For this review, use the dimensioned drawing (mm, ordinates from the lowest corner) and the shaded views. A direction names the side the tool comes from. Coordinates: 2 decimals unless noted, no trailing zeros. Write each loop counter-clockwise with the first axis right and the second up, starting at its lowest first coordinate (ties: lowest second). Pieces come first, ordered by that corner, then holes. Notation, with made-up numbers: (-1, -32.5) - (37, -32.5) arc R37 cw to (37, 5.5) - close; hole circle Ø3 at (-28.75, 53). An arc over 180 degrees is marked (long way). Put each result on its own line as item: value.
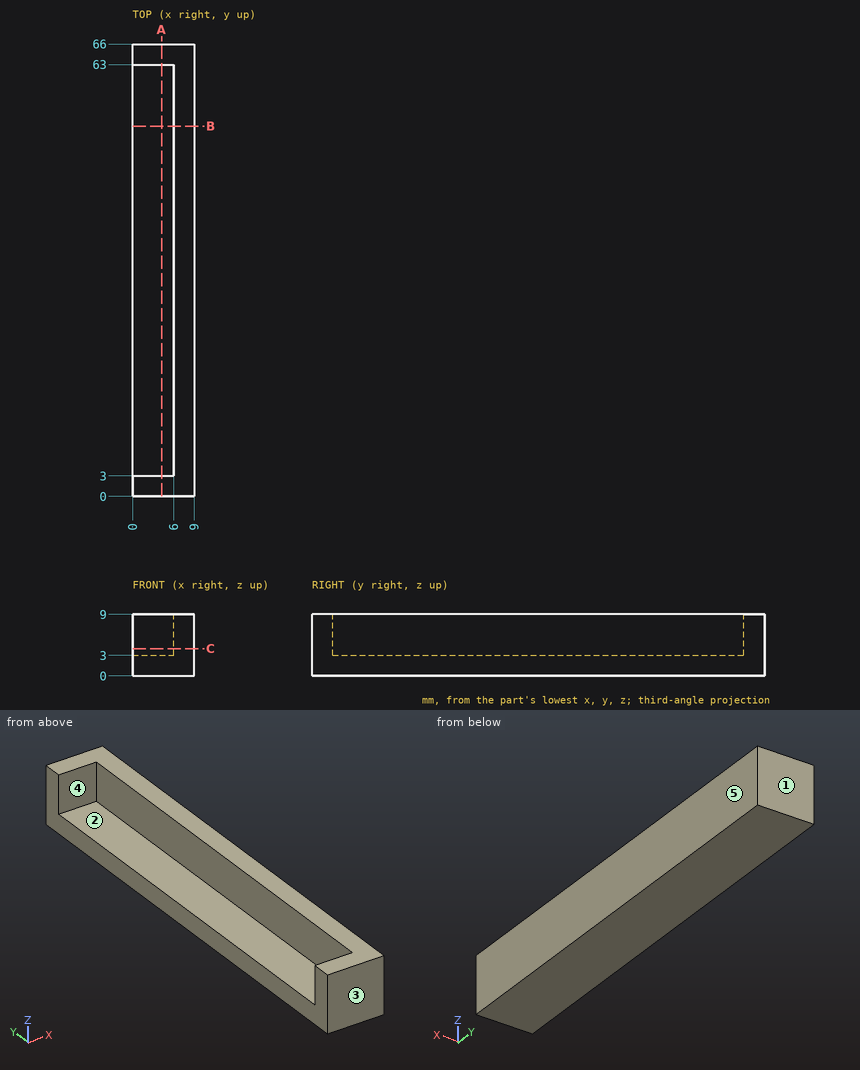
1. Machinability: for the marked faces 4 and 5, which of the approach directions +Z, -Z, +X, -X, +Y, -Y give a long, thin tool a straight path to every point of the face, cutting with its end or side? Answer none if there is none.
Determined:
face 4: +Z, -X
face 5: +Z, -Z, +X, +Y, -Y
2. The part is to be moulded in two halves that separate along Y. For the marked faces 1, 2 and 3, say which applies: +Y half, -Y half, draft (parallel to the pull), parting line (faces both ways), or undercut.
Determined:
face 1: +Y half
face 2: undercut
face 3: -Y half
3. Consider section B-B on y = 54. State the section outline as (x, z) points, plus the area to 3 significant figures.
Determined:
outline: (0, 0) - (9, 0) - (9, 9) - (6, 9) - (6, 3) - (0, 3) - close
area: 45.0 mm^2
4. For pin 1 Ø1.8 at (y, z) = (19, 6.5) entering from -X; pin 2 Ø5 at (x, y) = (2.5, 34.5) entering from +Z, all flat-tipped, find the tip position at first contact; note any pin that passes through.
Determined:
pin 1: stops at x = 6
pin 2: stops at z = 3
5. Consider section A-A on x = 4.25. State the section outline as (y, z) points, plus the area to 3 significant figures.
Determined:
outline: (0, 0) - (66, 0) - (66, 9) - (63, 9) - (63, 3) - (3, 3) - (3, 9) - (0, 9) - close
area: 234 mm^2
6. To check wall thickness, follow probe 1 along Y at (x, z) = (2.25, 3.25); probe 2 along X at (y, z) = (47, 4.5); probe 3 along Z at (x, y) = (1.75, 13.5). State the ranges of each line that lie inside material, in increasing order.
Determined:
probe 1: y = 0 to 3, 63 to 66
probe 2: x = 6 to 9
probe 3: z = 0 to 3
7. Consider section C-C on z = 4. State the section outline as (x, y) points, plus the area to 3 significant figures.
Determined:
outline: (0, 0) - (9, 0) - (9, 66) - (0, 66) - (0, 63) - (6, 63) - (6, 3) - (0, 3) - close
area: 234 mm^2
